Read the model definition and answer for the solid it produces. Units are mm, in the model's axes. A direction names the side the tool comes from. Give positions to 0.01 mm unless a question says otherwise; leave off trailing zeros. Order: outer loops, then holes, each group sorted by start corner. A loop starts at its lowest first (then second) coordinate and runs counter-clockwise, first axis right, second up. Notation, with made-up numbers: (-37, 78.5) -> (-25, 78.5) arc R37 ccw to (-25, 115.5) -> close; hole circle Ø4 at (-31.75, 22). An arc over 180 degrees is marked (long way). One line per item, written item: value. Start each with the question number.
from build123d import *

# Parameters (mm, degrees)
SKETCH4_R               = 1
SKETCH4_W               = 12.5
SKETCH4_H               = 22.5
CUT_EXTRUDE2_DEPTH      = 217.564078277
CUT_EXTRUDE3_REACH      = 196.487
SKETCH5_R               = 37.5
FILLET1_R               = 5
CUT_EXTRUDE4_REACH      = 218.564
CUT_EXTRUDE4_END_RADIUS = 56
SKETCH6_W               = 8.5
SKETCH6_H               = 8.5


with BuildPart() as part:
    # Sketch2 → Revolve1 (revolve)
    with BuildSketch(Plane.XY, mode=Mode.PRIVATE) as revolve1_sk:
        Polygon((35, -5), (40, -5), (60, 130), (60, 170), (0, 170), (0, 165), (56, 165), (56, 130), align=None)
    revolve(revolve1_sk.sketch.rotate(Axis((0, 170, 0), (0, -1, 0)), 90), axis=Axis((0, 170, 0), (0, -1, 0)))

    # Sketch4 → Cut-Extrude2 (cut, through all)
    with BuildSketch(Plane(origin=(60, 0, 0), x_dir=(0, 0, -1), z_dir=(1, 0, 0))):
        with Locations((0, 132.2)):
            Circle(SKETCH4_R)
        with Locations((0, 160)):
            Circle(SKETCH4_R)
        with Locations((0, 146.1)):
            Rectangle(SKETCH4_W, SKETCH4_H)
    extrude(amount=-CUT_EXTRUDE2_DEPTH, mode=Mode.SUBTRACT)

    # Sketch5 → Cut-Extrude3 (cut, up to next)
    with BuildSketch(Plane(origin=(0, 170, 0), x_dir=(1, 0, 0), z_dir=(0, 1, 0)), mode=Mode.PRIVATE) as cut_extrude3_sk1:
        with Locations(Location((0, 0, 0), (0, 0, 270))):
            Circle(SKETCH5_R)
    cut_extrude3_tool1 = extrude(cut_extrude3_sk1.sketch, amount=-CUT_EXTRUDE3_REACH, mode=Mode.PRIVATE) & part.part
    add(cut_extrude3_tool1.solids().sort_by_distance((0, 170, 0))[0], mode=Mode.SUBTRACT)

    # Fillet1
    fillet1_edges = [part.edges().sort_by_distance(p)[0] for p in [
        (0, 170, -60),
    ]]
    fillet(fillet1_edges, radius=FILLET1_R)

    # Cut-Extrude4: up to this cylinder (the profile starts outside it)
    cut_extrude4_end = Plane(origin=(0, 140.75, 0), z_dir=(0, 1, 0)) * Cylinder(CUT_EXTRUDE4_END_RADIUS, 550.128, mode=Mode.PRIVATE)
    # Sketch6 → Cut-Extrude4 (cut, up to the surface)
    with BuildSketch(Plane.XY.offset(60), mode=Mode.PRIVATE) as cut_extrude4_sk1:
        with Locations((0, 140.75)):
            Rectangle(SKETCH6_W, SKETCH6_H)
    cut_extrude4_tool1 = extrude(cut_extrude4_sk1.sketch, amount=-CUT_EXTRUDE4_REACH, mode=Mode.PRIVATE) - cut_extrude4_end
    add(cut_extrude4_tool1.solids().sort_by_distance((0, 140.75, 60))[0], mode=Mode.SUBTRACT)


solid = part.part
Item 1: Find section D-D on y = 31.5. Write down the section's boundary in (x, z).
Item 2: For a pull along Z with two mould halves and no side action, classify faces 1 (the cylindrical face through (-50.59, 147.74, 32.26)), 2 (the flat face through (0, 145, 58)), 3 (the flat face through (58, 146, 6.25)) as +Z half, -Z half, draft (parallel to the pull), parting line (faces both ways), or undercut.
Item 3: Find section B-B on z = 3. Count the separate pieces of the cut face and the enclosed holes in it, then the cut area to 3 significant figures.
Item 4: Find section C-C on y = 63. Write down the section's boundary in (x, z).
Item 5: Flat-ended cylindrical pins translate along their axes: pin 1 (10 mm diameter, centred on y = 94.5, z = 34, fed in from -X); pin 2 (1 mm diameter, centred on x = -37.5, y = 90.5, fed in from +Z); pin 3 (3 mm diameter, centred on y = 149, z = 21.5, fed in from +X); pin 4 (1.8 mm diameter, centred on y = 160, z = 0, fed in from +X). Find the tip coordinate at first contact, or state that the pin passes through.
Item 6: A tool of negligible diameter and unlimited length cuts with its end or side. For faces 4 (the flat face through (-58, 157.35, 0)), 5 (the flat face through (37, 165, -12)), 6 (the flat face through (-4.25, 141, 58)), from which of +Z, -Z, +X, -X, +Y, -Y can it reach the whole face along a straight path? Write none if from no direction.
Item 7: Find the intervals of material crossed by line 1 (Z direction, x = -1, y = 154); line 2 (X direction, y = 141.5, z = -51.5); line 3 (Z direction, x = -31.5, y = 41), in increasing order. Write a range as from..to.
Item 8: Find section A-A on x = 0. Write down the section's boundary in (y, z), then the cut area to 3 significant figures.
Checks:
1. outline: circle Ø90.81 at (0, 0); hole circle Ø81.36 at (0, 0)
2. face 1: parting line
2. face 2: draft
2. face 3: undercut
3. separate pieces: 4
3. enclosed holes: 0
3. area: 1,530 mm2
4. outline: circle Ø100.15 at (0, 0); hole circle Ø91.16 at (0, 0)
5. pin 1: x = -46.55
5. pin 2: z = 39.55
5. pin 3: x = 56.57
5. pin 4: through
6. face 4: +X, -X
6. face 5: none
6. face 6: +Z
7. line 1: -59.99..-55.99, 55.99..59.99
7. line 2: -30.79..-21.99, 21.99..30.79
7. line 3: -34.63..-28.02, 28.02..34.63
8. outline: (-5, -40) -> (130, -60) -> (165, -60) arc R5 ccw to (170, -55) -> (170, -37.5) -> (165, -37.5) -> (165, -56) -> (130, -56) -> (-5, -35) -> close; (-5, 35) -> (130, 56) -> (136.5, 56) -> (136.5, 60) -> (130, 60) -> (-5, 40) -> close; (145, 56) -> (165, 56) -> (165, 37.5) -> (170, 37.5) -> (170, 55) arc R5 ccw to (165, 60) -> (145, 60) -> close
8. area: 1,680 mm2
